```python
from build123d import *

# Parameters (mm, degrees)
BOSS_EXTRUDE1_DEPTH = 40
SKETCH3_R           = 5
CUT_EXTRUDE1_DEPTH  = 40
SKETCH4_R           = 2.5
CUT_EXTRUDE2_DEPTH  = 40


with BuildPart() as part:
    # Sketch2 → Boss-Extrude1 (new body)
    with BuildSketch(Plane.XY):
        with BuildLine():
            Line((0, 2), (0, 40))
            Line((0, 40), (5, 40))
            Line((5, 40), (5, 7))
            ThreePointArc((5, 7), (5.585786438, 5.585786438), (7, 5))
            Line((7, 5), (40, 5))
            Line((40, 5), (40, 0))
            Line((40, 0), (2, 0))
            ThreePointArc((2, 0), (0.585786438, 0.585786438), (0, 2))
        make_face()
    extrude(amount=BOSS_EXTRUDE1_DEPTH)

    # Sketch3 → Cut-Extrude1 (cut)
    with BuildSketch(Plane(origin=(5, 0, 0), x_dir=(0, 0, -1), z_dir=(1, 0, 0))):
        with Locations((-20, 25)):
            Circle(SKETCH3_R)
    extrude(amount=-CUT_EXTRUDE1_DEPTH, mode=Mode.SUBTRACT)

    # Sketch4 → Cut-Extrude2 (cut)
    with BuildSketch(Plane(origin=(0, 5, 0), x_dir=(1, 0, 0), z_dir=(0, 1, 0))):
        with Locations((25, -10)):
            Circle(SKETCH4_R)
        with Locations((25, -30)):
            Circle(SKETCH4_R)
    extrude(amount=-CUT_EXTRUDE2_DEPTH, mode=Mode.SUBTRACT)


solid = part.part
```
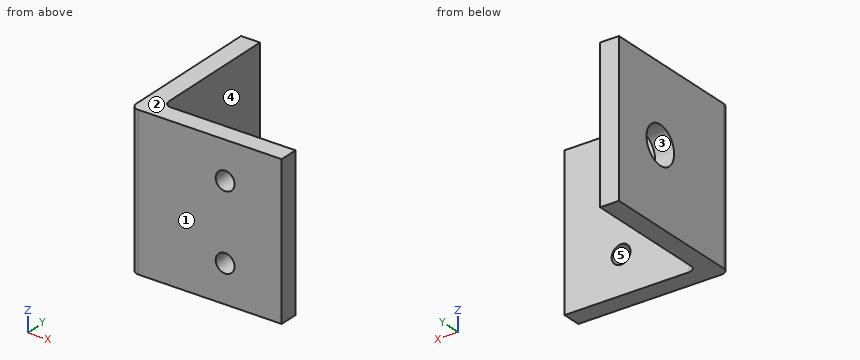
Work out the finished part from the listing and answer in its coordinate system (mm). Face numbers are marked on the shaded views. A direction names the side the tool comes from. Round coordinates to 2 decimals unless told otherwise and drop trailing zeros. Write each loop counter-clockwise with the first axis right and the second up, starting at its lowest first coordinate (ties: lowest second). Pieces come first, ordered by that corner, then holes.
1) Which of the six approach directions +Z, -Z, +X, -X, +Y, -Y give full straight-line access (tool end or side, diameter ignored) to the marked faces 4 and 5?
2) A cutting plane is placed at D-D on z = 6.5. Determine the outline of the cut face in (x, y).
3) A cutting plane is placed at B-B on z = 20. Determine the outline of the cut face in (x, y), and give its area (3 significant figures).
4) A cutting plane is placed at C-C on y = 25. Determine the outline of the cut face in (x, z), and give its area (3 significant figures).
5) Consider probe 1 along Z at (x, y) = (25, 2.55); probe 2 along Y at (x, z) = (3, 20); probe 3 along X at (y, z) = (1.85, 30). Determine where each line is inside the solid, lowest interval first.
6) Flat-ended cylindrical pins translate along their axes: P1, Ø16.5, axis at x = 28.5, z = 17.5, coming from the +Y side; P2, Ø13, axis at y = 25, z = 20, coming from the +X side; P3, Ø5, axis at x = 20, z = 15, coming from the -Y side; P4, Ø10, axis at x = 33, y = 13, coming from the +Z side. Find the tip coordinate at first contact, or state that the pin passes through.
7) Determine the mould class of the marked faces 1, 2 and 3 for opening direction Z: pulls with the +Z half, pulls with the -Z half, needs draft (parallel to the pull), parting line crosses it, or undercut.
8) A cutting plane is placed at A-A on x = 25. Determine the outline of the cut face in (y, z).
Entries:
1. face 4: +Z, -Z, +X, +Y
1. face 5: +Y, -Y
2. outline: (0, 2) arc R2 ccw to (2, 0) - (40, 0) - (40, 5) - (7, 5) arc R2 cw to (5, 7) - (5, 40) - (0, 40) - close
3. outline: (0, 2) arc R2 ccw to (2, 0) - (40, 0) - (40, 5) - (7, 5) arc R2 cw to (5, 7) - (5, 20) - (0, 20) - close; (0, 30) - (5, 30) - (5, 40) - (0, 40) - close
3. area: 325 mm2
4. outline: (0, 0) - (5, 0) - (5, 15) - (0, 15) - close; (0, 25) - (5, 25) - (5, 40) - (0, 40) - close
4. area: 150 mm2
5. probe 1: z = 0 to 7.5, 12.5 to 27.5, 32.5 to 40
5. probe 2: y = 0 to 20, 30 to 40
5. probe 3: x = 0.01 to 22.5, 27.5 to 40
6. P1: stops at y = 5
6. P2: stops at x = 5
6. P3: stops at y = 0
6. P4: passes through
7. face 1: needs draft
7. face 2: pulls with the +Z half
7. face 3: undercut
8. outline: (0, 0) - (5, 0) - (5, 7.5) - (0, 7.5) - close; (0, 12.5) - (5, 12.5) - (5, 27.5) - (0, 27.5) - close; (0, 32.5) - (5, 32.5) - (5, 40) - (0, 40) - close
